from build123d import *

# Parameters (mm, degrees)
BOSS_EXTRUDE1_DEPTH = 74.5
FILLET1_R           = 7
FILLET2_R           = 2
FILLET3_R           = 1.5
FILLET4_R           = 3
SKETCH3_R           = 5.5
SKETCH3_R_2         = 2
SKETCH3_W           = 31
SKETCH3_H           = 23
CUT_EXTRUDE1_DEPTH  = 1.5
FILLET5_R           = 2
BOSS_EXTRUDE3_DEPTH = 1.5


with BuildPart() as part:
    # Sketch1 → Boss-Extrude1 (new body)
    with BuildSketch(Plane(origin=(0, 0, 0), x_dir=(0, 0, -1), z_dir=(1, 0, 0))):
        Polygon((-20.859650045, -2.828427125), (0, -2.828427125), (24.536605307, -2.828427125), (24.536605307, 0.171572875), (3, 0.171572875), (24.536605307, 21.708178182), (14.106780285, 32.138003205), (-10.429825023, 7.601397898), align=None)
        Polygon((19.339370465, 24.996224715), (18.879751058, 24.536605307), (21.708178182, 21.708178182), (0, 0), (-2.828427125, 2.828427125), (-3.288046533, 2.368807717), (-4.171930009, 3.252691193), (-3.712310601, 3.712310601), (-7.954951288, 7.954951288), (13.753226894, 29.663129471), (17.995867581, 25.420488784), (18.455486989, 25.880108191), align=None, mode=Mode.SUBTRACT)
    extrude(amount=BOSS_EXTRUDE1_DEPTH)

    # Fillet1
    fillet1_edges = [part.edges().sort_by_distance(p)[0] for p in [
        (37.25, -2.828427125, 20.859650045),
    ]]
    fillet(fillet1_edges, radius=FILLET1_R)

    # Fillet2
    fillet2_edges = [part.edges().sort_by_distance(p)[0] for p in [
        (37.25, 32.138003205, -14.106780285),
        (37.25, 21.708178182, -24.536605307),
        (37.25, 29.663129471, -13.753226894),
        (37.25, 7.954951288, 7.954951288),
        (37.25, 0, 0),
        (37.25, 21.708178182, -21.708178182),
    ]]
    fillet(fillet2_edges, radius=FILLET2_R)

    # Fillet3
    fillet3_edges = [part.edges().sort_by_distance(p)[0] for p in [
        (37.25, -2.828427125, -24.536605307),
        (37.25, 0.171572875, -24.536605307),
    ]]
    fillet(fillet3_edges, radius=FILLET3_R - 0.0001)  # a hair under: the kernel refuses the full size

    # Fillet4
    fillet4_edges = [part.edges().sort_by_distance(p)[0] for p in [
        (37.25, 0.171572875, -3),
    ]]
    fillet(fillet4_edges, radius=FILLET4_R)

    # Sketch3 → Cut-Extrude1 (cut)
    with BuildSketch(Plane(origin=(0, 9.01561146, 9.01561146), x_dir=(1, 0, 0), z_dir=(0, 0.7071067811865475, 0.7071067811865476))):
        with Locations(Location((11, 19.35, 0), (0, 0, 270))):
            Circle(SKETCH3_R)
        with Locations(Location((11, 3.85, 0), (0, 0, 270))):
            Circle(SKETCH3_R_2)
        with Locations((34.5, 15.35)):
            Rectangle(SKETCH3_W, SKETCH3_H)
    extrude(amount=-CUT_EXTRUDE1_DEPTH, mode=Mode.SUBTRACT)

    # Fillet5
    fillet5_edges = [part.edges().sort_by_distance(p)[0] for p in [
        (19, 11.207642482, 5.762920267),
        (19, 27.471098449, -10.500535701),
        (50, 27.471098449, -10.500535701),
        (50, 11.207642482, 5.762920267),
    ]]
    fillet(fillet5_edges, radius=FILLET5_R)

    # Sketch4 → Boss-Extrude3 (add)
    with BuildSketch(Plane.ZY):
        with BuildLine():
            Line((-23.036605307, -2.828427125), (3.960155108, -2.828427125))
            ThreePointArc((3.960155108, -2.828427125), (10.427311836, 1.492788849), (8.909902577, 9.121320344))
            Line((8.909902577, 9.121320344), (-12.692566722, 30.723789643))
            ThreePointArc((-12.692566722, 30.723789643), (-14.106780285, 31.30957608), (-15.520993847, 30.723789643))
            Line((-15.520993847, 30.723789643), (-23.122391745, 23.122391745))
            ThreePointArc((-23.122391745, 23.122391745), (-23.708178182, 21.708178182), (-23.122391745, 20.29396462))
            Line((-23.122391745, 20.29396462), (-8.121320344, 5.292893219))
            ThreePointArc((-8.121320344, 5.292893219), (-7.47100209, 2.023522578), (-10.242640687, 0.171572875))
            Line((-10.242640687, 0.171572875), (-23.036605307, 0.171572875))
            ThreePointArc((-23.036605307, 0.171572875), (-24.097265479, -0.267766953), (-24.536605307, -1.328427125))
            ThreePointArc((-24.536605307, -1.328427125), (-24.097265479, -2.389087297), (-23.036605307, -2.828427125))
        make_face()
    extrude(amount=BOSS_EXTRUDE3_DEPTH)


solid = part.part
Verification items for the finished model (mm, model axes). A direction names the side the tool comes from. Coordinates: 2 decimals unless noted, no trailing zeros. Order: outer loops, then holes, each group sorted by start corner. A loop starts at its lowest first (then second) coordinate and runs counter-clockwise, first axis right, second up.
1. Set-up check for faces 4 (the face through (19.57, 11.625, 5.33)), 5 (the face through (37.03, 12.9, -15.73)), 6 (the face through (49.4, 27.06, -10.1)), 7 (the face through (37.77, 21.69, -20.88)): record each of +Z, -Z, +X, -X, +Y, -Y from which the full face is reachable in a straight line by a thin tool's end or side.
Results found:
face 4: +Y
face 5: -Z, +X, -X
face 6: +Z
face 7: +X
2. Scan lines: line 1 (Y direction, x = 39, z = -20.5); line 2 (Y direction, x = 50, z = -15.5); line 3 (X direction, y = 18.5, z = -6). Record each from-to range of solid material in increasing order.
Results found:
line 1: y = -2.83 to 0.17, 17.67 to 20.54, 22.88 to 25.74
line 2: y = -2.83 to 0.17, 12.67 to 15.5, 27.92 to 30.74
line 3: x = -1.5 to 0
3. Go/stop test with flat-tipped pins: pin 1 Ø6 at (x, y) = (62.5, 24) entering from -Z; pin 2 Ø3 at (x, z) = (38, -19) entering from +Y. Record where each tip stops, or that it passes through.
Results found:
pin 1: stops at z = -23.71
pin 2: stops at y = 28.74
4. Release check for a two-part mould opening along Y. For faces 1 (the face through (37.772, 7.977, 7.126)), 2 (the face through (37, -2.828, -10)), 3 (the face through (-0.74, 1.386, 10.382)) record: +Y half, -Y half, draft (parallel to the pull), parting line (faces both ways), or undercut.
Results found:
face 1: undercut
face 2: -Y half
face 3: parting line
5. Sectioned sample at B-B, the plane y = 22. Give the number of separate pieces and of enclosed holes in the cut face, and give its area (3 significant figures).
Results found:
separate pieces: 3
enclosed holes: 0
area: 309 mm2
6. Sectioned sample at A-A, the plane z = -14. Record the cut outline in (x, y), and give its area (3 significant figures).
Results found:
outline: (-1.5, -2.83) - (74.5, -2.83) - (74.5, 0.17) - (-1.5, 0.17) - close; (-1.5, 11.17) - (74.5, 11.17) - (74.5, 14) - (0, 14) - (0, 28.82) - (74.5, 28.82) - (74.5, 31.31) - (-1.5, 31.31) - close
area: 654 mm2
